Read the model definition and answer for the solid it produces. Units are mm, in the model's axes. Face numbers are marked on the shaded views. A direction names the side the tool comes from. Round coordinates to 2 decimals unless told otherwise and drop trailing zeros. Loops run counter-clockwise (first coordinate to the right, second up) from the corner with the lowest first, then second, coordinate; pieces in that order, holes last. Notation, with made-up numbers: (37.25, 50.5) - (48.25, 50.5) arc R21 cw to (48.25, 55.5) - close; hole circle Ø5 at (-11, -37.75). An arc over 180 degrees is marked (long way). Use CSV: the item, a comma, the result in double quotes. Start each with the question number.
1. Find section B-B (z = 3.25). Give the vertices of the cut face in (x, y).
2. Find section D-D (z = -0.75). Give the vertices of the cut face in (x, y).
3. Find section A-A (x = 0). Give the vertices of the cut face in (y, z).
4. Find section C-C (y = 0.5). Give the vertices of the cut face in (x, z), and give its area (3 significant figures).
5. A tool of negligible diameter and unlimited length cuts with its end or side. For the marked faces 5 and 6, from which of +Z, -Z, +X, -X, +Y, -Y can it reach the whole face along a straight path? Write none if from no direction.
6. Given pin 1 Ø3 at (x, z) = (0, 3) entering from -Y, flat-ended and moving along its own axis, determine where the tip first touches the part or whether it passes through.
7. Determine the mould class of the marked faces 1, 2, 3 and 4 for opening direction X: +X half, -X half, draft (parallel to the pull), parting line (faces both ways), or undercut.
8. Consider line 1 along X through (y, z) = (1.2, -5); line 2 along X through (y, z) = (1.35, -3.25); line 3 along Z through (x, y) = (0.25, 0.5). Determine where each line is inside the solid, lowest interval first.
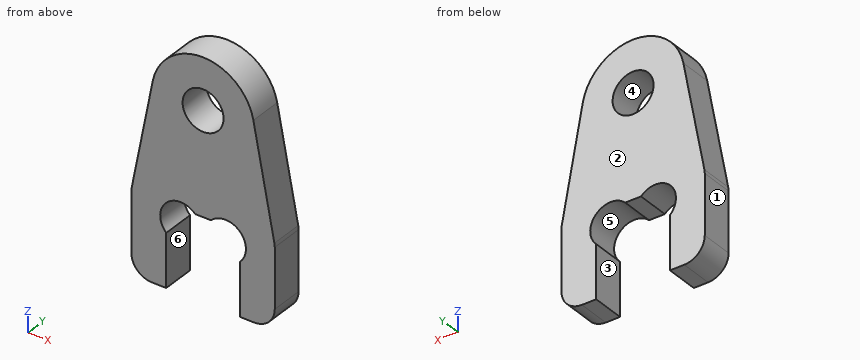
from build123d import *

# Parameters (mm, degrees)
SKETCH1_W               = 7
SKETCH1_H               = 12
BOSS_EXTRUDE1_DEPTH     = 1.6
SKETCH3_W               = 3.6
SKETCH3_H               = 4
CUT_EXTRUDE2_DEPTH      = 8.128113355
SKETCH4_R               = 1
CUT_EXTRUDE3_DEPTH      = 10
CUT_EXTRUDE4_DEPTH      = 8.128113355
CUT_EXTRUDE4_DEPTH_BACK = 8.128113355
FILLET1_R               = 1
CUT_EXTRUDE5_DEPTH      = 8.128113355


with BuildPart() as part:
    # Sketch1 → Boss-Extrude1 (new body)
    with BuildSketch(Plane(origin=(0, 0, 0), x_dir=(1, 0, 0), z_dir=(0, 1, 0))):
        Rectangle(SKETCH1_W, SKETCH1_H)
    extrude(amount=BOSS_EXTRUDE1_DEPTH)

    # Sketch3 → Cut-Extrude2 (cut, through all)
    with BuildSketch(Plane.XZ):
        with Locations((0, -4)):
            Rectangle(SKETCH3_W, SKETCH3_H)
    extrude(amount=-CUT_EXTRUDE2_DEPTH, mode=Mode.SUBTRACT)

    # Sketch4 → Cut-Extrude3 (cut)
    with BuildSketch(Plane(origin=(0, 1.6, 0), x_dir=(1, 0, 0), z_dir=(0, 1, 0))):
        with Locations(Location((0, -3, 0), (0, 0, 270))):
            Circle(SKETCH4_R)
    extrude(amount=-CUT_EXTRUDE3_DEPTH, mode=Mode.SUBTRACT)

    # Sketch5 → Cut-Extrude4 (cut, two sides: drawn at the far end of the back side and taken through both)
    with BuildSketch(Plane(origin=(0, 1.6, 0), x_dir=(1, 0, 0), z_dir=(0, 1, 0)).offset(-CUT_EXTRUDE4_DEPTH_BACK)):
        with BuildLine():
            Line((2.455625625, -3.468937938), (3.5, 2))
            Line((3.5, 2), (6.178310216, -2.368643633))
            Line((6.178310216, -2.368643633), (0.801322839, -12.436782797))
            Line((0.801322839, -12.436782797), (-8.05270341, -5.5))
            Line((-8.05270341, -5.5), (-3.5, 2))
            Line((-3.5, 2), (-2.455625625, -3.468937938))
            ThreePointArc((-2.455625625, -3.468937938), (0, -5.5), (2.455625625, -3.468937938))
        make_face()
    extrude(amount=CUT_EXTRUDE4_DEPTH + CUT_EXTRUDE4_DEPTH_BACK, mode=Mode.SUBTRACT)

    # Fillet1
    fillet1_edges = [part.edges().sort_by_distance(p)[0] for p in [
        (3.5, 0.8, -2),
        (-3.5, 0.8, -2),
        (-3.5, 0.8, -6),
        (3.5, 0.8, -6),
    ]]
    fillet(fillet1_edges, radius=FILLET1_R)

    # Sketch8 → Cut-Extrude5 (cut, through all)
    with BuildSketch(Plane(origin=(0, 1.6, 0), x_dir=(1, 0, 0), z_dir=(0, 1, 0))):
        with BuildLine():
            Line((1.8, 3.414213562), (0.385786438, 2))
            ThreePointArc((0.385786438, 2), (1.8, 2), (1.8, 3.414213562))
        make_face()
        with BuildLine():
            Line((-1.8, 3.414213562), (-0.385786438, 2))
            ThreePointArc((-0.385786438, 2), (-1.8, 2), (-1.8, 3.414213562))
        make_face()
    extrude(amount=-CUT_EXTRUDE5_DEPTH, mode=Mode.SUBTRACT)


solid = part.part
Filled sheet:
1,outline,"(-2.5, 0) - (-0.97, 0) - (-0.97, 1.6) - (-2.5, 1.6) - close; (0.97, 0) - (2.5, 0) - (2.5, 1.6) - (0.97, 1.6) - close"
2,outline,"(-3.26, 0) - (3.26, 0) - (3.26, 1.6) - (-3.26, 1.6) - close"
3,outline,"(0, -2) - (1.6, -2) - (1.6, 2) - (0, 2) - close; (0, 4) - (1.6, 4) - (1.6, 5.5) - (0, 5.5) - close"
4,outline,"(-3.5, -5) arc R1 ccw to (-2.5, -6) - (-1.8, -6) - (-1.8, -3.41) arc R1 cw to (-0.39, -2) - (0.39, -2) arc R1 cw to (1.8, -3.41) - (1.8, -6) - (2.5, -6) arc R1 ccw to (3.5, -5) - (3.5, -2.09) arc R1 ccw to (3.48, -1.91) - (2.46, 3.47) arc R2.5 ccw to (-2.46, 3.47) - (-3.48, -1.91) arc R1 ccw to (-3.5, -2.09) - close; hole circle Ø2 at (0, 3)"
4,area,"48.9 mm²"
5,face 5,"+Y, -Y"
5,face 6,"-Z, +Y, -Y"
6,pin 1,"stops at y = 0"
7,face 1,"-X half"
7,face 2,"draft"
7,face 3,"undercut"
7,face 4,"undercut"
8,line 1,"x = -3.5 to -1.8, 1.8 to 3.5"
8,line 2,"x = -3.5 to -1.93, 1.93 to 3.5"
8,line 3,"z = -2 to 2.03, 3.97 to 5.49"
